```python
from build123d import *

# Parameters (mm, degrees)
F0_R     = 10
F1_DEPTH = 6
F2_SIZE  = 5
F4_DEPTH = 4
F5_R     = 1.625
F6_DEPTH = 5


with BuildPart() as f1:
    # F0 (on Top) → F1 (new body)
    with BuildSketch(Plane.XY):
        Circle(F0_R)
    extrude(amount=F1_DEPTH)

    # F2
    f2_edges = [f1.edges().sort_by_distance(p)[0] for p in [
        (-10, 0, 6),
    ]]
    chamfer(f2_edges, length=F2_SIZE)

    # F3 (on face) → F4 (cut)
    with BuildSketch(Plane.XY.offset(6)):
        Polygon((0.150565, -4.616347), (4.073156, -2.177781), (3.922592, 2.438566), (-0.150565, 4.616347), (-4.073156, 2.177781), (-3.922592, -2.438566), align=None)
    extrude(amount=-F4_DEPTH, mode=Mode.SUBTRACT)

    # F5 (on Top) → F6 (cut)
    with BuildSketch(Plane.XY):
        Circle(F5_R)
    extrude(amount=F6_DEPTH, mode=Mode.SUBTRACT)


solid = f1.part
```
Can you work these out from the model? Positions are in its coordinate system, mm. A direction names the side the tool comes from. Round coordinates to 2 decimals unless told otherwise and drop trailing zeros. Loops run counter-clockwise (first coordinate to the right, second up) from the corner with the lowest first, then second, coordinate; pieces in that order, holes last. Notation, with made-up numbers: (32, -20.75) -> (53, -20.75) arc R10 cw to (53, -8.75) -> close; hole circle Ø11 at (46.25, 49.25). An arc over 180 degrees is marked (long way). One line per item, written item: value. Start each with the question number.
1. If we mould it in two halves opening along Y, with no side actions, what happens to faces 1 (the conical face through (-4.16, -3.19, 5.76)), 2 (the flat face through (2, 0, 0)), 3 (the cylindrical face through (-1.29, -0.99, 0.99))? For each: pulls with the +Y half, pulls with the -Y half, needs draft (parallel to the pull), parting line crosses it, or undercut.
2. If I drill on probe 1 along Y at (x, z) = (0, 0.5) (3 decimals); probe 2 along X at (y, z) = (0, 1.1) (3 decimals); probe 3 along X at (y, z) = (1.25, 3.7), over which ranges is the centre line in solid material (lowest first)?
3. For faces 4 (the cylindrical face through (-2.17, -9.76, 0.49)), 5 (the flat face through (2.084, -3.414, 4.028)), which set-ups out of +Z, -Z, +X, -X, +Y, -Y let a thin tool reach every point of the face, with its end or its side?
4. For pin 1 (6 mm diameter, centred on x = 6, y = 8, fed in from +Z); pin 2 (3 mm diameter, centred on x = 4.5, z = 3.5, fed in from +Y); pin 3 (1 mm diameter, centred on y = 2, z = 5, fed in from +X), each with a flat end and sliding along its axis, tell me the tip position at first contact or that it passes through.
5. If we section it at A-A, the plane z = 2.3: Write out the boundary of the cut face in (x, y), then the cut area to 3 significant figures.
6. If we section it at C-C, the plane z = 5.5: Write out the boundary of the cut face in (x, y).
7. If we section it at B-B, the plane y = 0: Write out the boundary of the cut face in (x, z) (3 decimals), then the cut area to 3 significant figures.
8. If we section it at D-D, the plane z = 0.5: Write out the boundary of the cut face in (x, y) (3 decimals), then the cut area to 3 significant figures.
Calculated:
1. face 1: parting line crosses it
1. face 2: needs draft
1. face 3: undercut
2. probe 1: y = -10 to -1.625, 1.625 to 10
2. probe 2: x = -9.9 to -1.625, 1.625 to 9.9
2. probe 3: x = -7.19 to -4.04, 3.96 to 7.19
3. face 4: +Z, -Z
3. face 5: +Z
4. pin 1: stops at z = 4
4. pin 2: stops at y = 7.97
4. pin 3: stops at x = 6.21
5. outline: circle Ø17.4 at (0, 0); hole (-4.07, 2.18) -> (-3.92, -2.44) -> (0.15, -4.62) -> (4.07, -2.18) -> (3.92, 2.44) -> (-0.15, 4.62) -> close
5. area: 182 mm²
6. outline: circle Ø11 at (0, 0); hole (-4.07, 2.18) -> (-3.92, -2.44) -> (0.15, -4.62) -> (4.07, -2.18) -> (3.92, 2.44) -> (-0.15, 4.62) -> close
7. outline: (-10, 0) -> (-1.625, 0) -> (-1.625, 2) -> (-4.002, 2) -> (-4.002, 6) -> (-5, 6) -> (-10, 1) -> close; (1.625, 0) -> (10, 0) -> (10, 1) -> (5, 6) -> (4.002, 6) -> (4.002, 2) -> (1.625, 2) -> close
7. area: 56.5 mm²
8. outline: circle Ø20 at (0, 0); hole circle Ø3.25 at (0, 0)
8. area: 306 mm²
